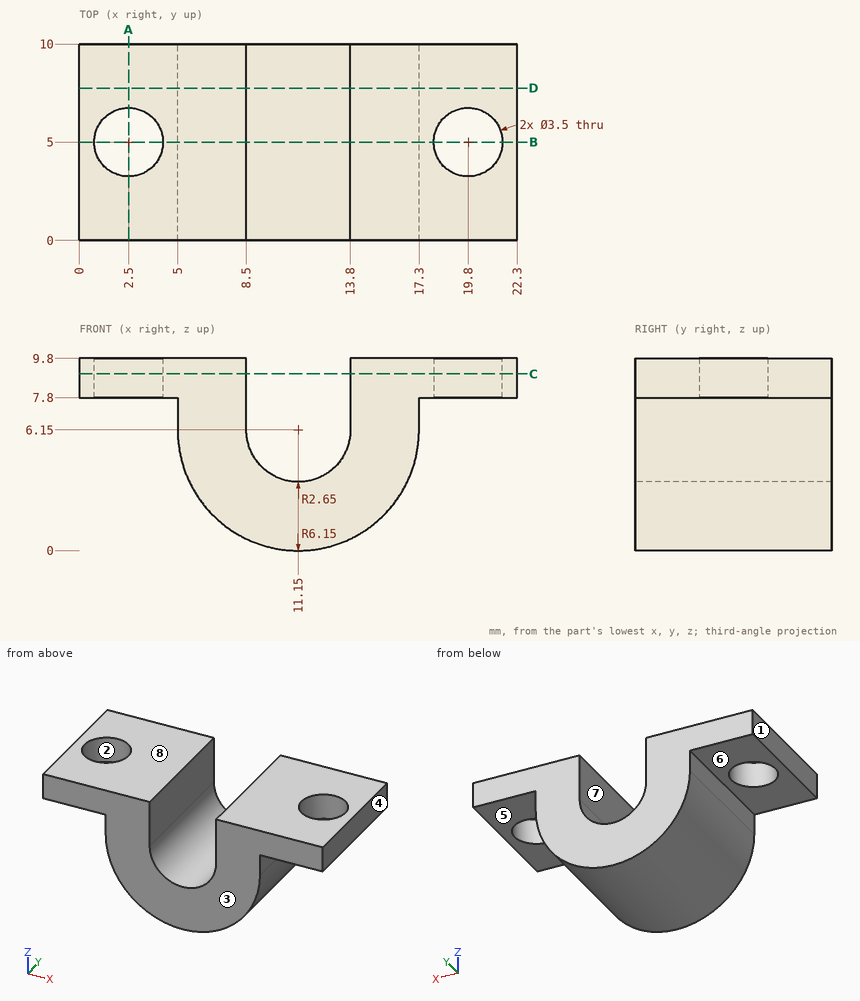
Could you check a few things on this drawing? It's one solid part, dimensions in mm from its lowest x, y, z. A direction names the side the tool comes from. Give positions to 0.01 mm unless a question says otherwise; leave off trailing zeros. Order: outer loops, then holes, each group sorted by start corner. A loop starts at its lowest first (then second) coordinate and runs counter-clockwise, first axis right, second up. Notation, with made-up numbers: (56, -36) - (71, -36) arc R9 cw to (71, -20) - close; hole circle Ø11 at (-15, -33.75). An arc over 180 degrees is marked (long way). Answer as a JSON object with one key per item and string values. Group by question number.
Item 1: For P1, Ø2.5, axis at x = 21, y = 4, coming from the -Z side; P2, Ø1.3, axis at y = 7, z = 7, coming from the -X side; P3, Ø1, axis at y = 1, z = 3, coming from the -X side, each with a flat end and sliding along its axis, tell me the tip position at first contact or that it passes through.
Item 2: If we section it at D-D on y = 7.75: Please give me the cut outline in (x, z).
Item 3: Please list where these lines run through material, in increasing order: probe 1 along Y at (x, z) = (19.8, 8.7); probe 2 along X at (y, z) = (2.75, 6.5); probe 3 along X at (y, z) = (9.25, 8).
Item 4: If we section it at B-B on y = 5: Please give me the cut outline in (x, z), and give its area (3 significant figures).
Item 5: If we section it at C-C on z = 9: Please give me the cut outline in (x, y).
Item 6: If we section it at A-A on x = 2.5: Please give me the cut outline in (y, z), and give its area (3 significant figures).
Item 7: If we mould it in two halves opening along X, with no side actions, what happens to the marked faces 1, 2 and 3? For each: pulls with the +X half, pulls with the -X half, needs draft (parallel to the pull), parting line crosses it, or undercut.
Item 8: Which directions (+Z, -Z, +X, -X, +Y, -Y) give clear straight access to the entire face, cutting with the end or side of a thin tool? Please do the marked faces 4, 5, 6, 7 and 8.
Result set:
{
 "1": {"P1": "z = 7.8", "P2": "x = 5", "P3": "x = 5.6"},
 "2": {"outline": "(0, 7.8) - (5, 7.8) - (5, 6.15) arc R6.15 ccw to (17.3, 6.15) - (17.3, 7.8) - (22.3, 7.8) - (22.3, 9.8) - (13.8, 9.8) - (13.8, 6.15) arc R2.65 cw to (8.5, 6.15) - (8.5, 9.8) - (0, 9.8) - close"},
 "3": {"probe 1": "0 to 3.25, 6.75 to 10", "probe 2": "5 to 8.5, 13.8 to 17.3", "probe 3": "0 to 8.5, 13.8 to 22.3"},
 "4": {"outline": "(0, 7.8) - (0.75, 7.8) - (0.75, 9.8) - (0, 9.8) - close; (4.25, 7.8) - (5, 7.8) - (5, 6.15) arc R6.15 ccw to (17.3, 6.15) - (17.3, 7.8) - (18.05, 7.8) - (18.05, 9.8) - (13.8, 9.8) - (13.8, 6.15) arc R2.65 cw to (8.5, 6.15) - (8.5, 9.8) - (4.25, 9.8) - close; (21.55, 7.8) - (22.3, 7.8) - (22.3, 9.8) - (21.55, 9.8) - close", "area": "79.9 mm²"},
 "5": {"outline": "(0, 0) - (8.5, 0) - (8.5, 10) - (0, 10) - close; (13.8, 0) - (22.3, 0) - (22.3, 10) - (13.8, 10) - close; hole circle Ø3.5 at (2.5, 5); hole circle Ø3.5 at (19.8, 5)"},
 "6": {"outline": "(0, 7.8) - (3.25, 7.8) - (3.25, 9.8) - (0, 9.8) - close; (6.75, 7.8) - (10, 7.8) - (10, 9.8) - (6.75, 9.8) - close", "area": "13.0 mm²"},
 "7": {"face 1": "pulls with the -X half", "face 2": "undercut", "face 3": "needs draft"},
 "8": {"face 4": "+Z, -Z, +X, +Y, -Y", "face 5": "-Z, +X, +Y, -Y", "face 6": "-Z, -X, +Y, -Y", "face 7": "+Z, +Y, -Y", "face 8": "+Z, +X, -X, +Y, -Y"}
}
